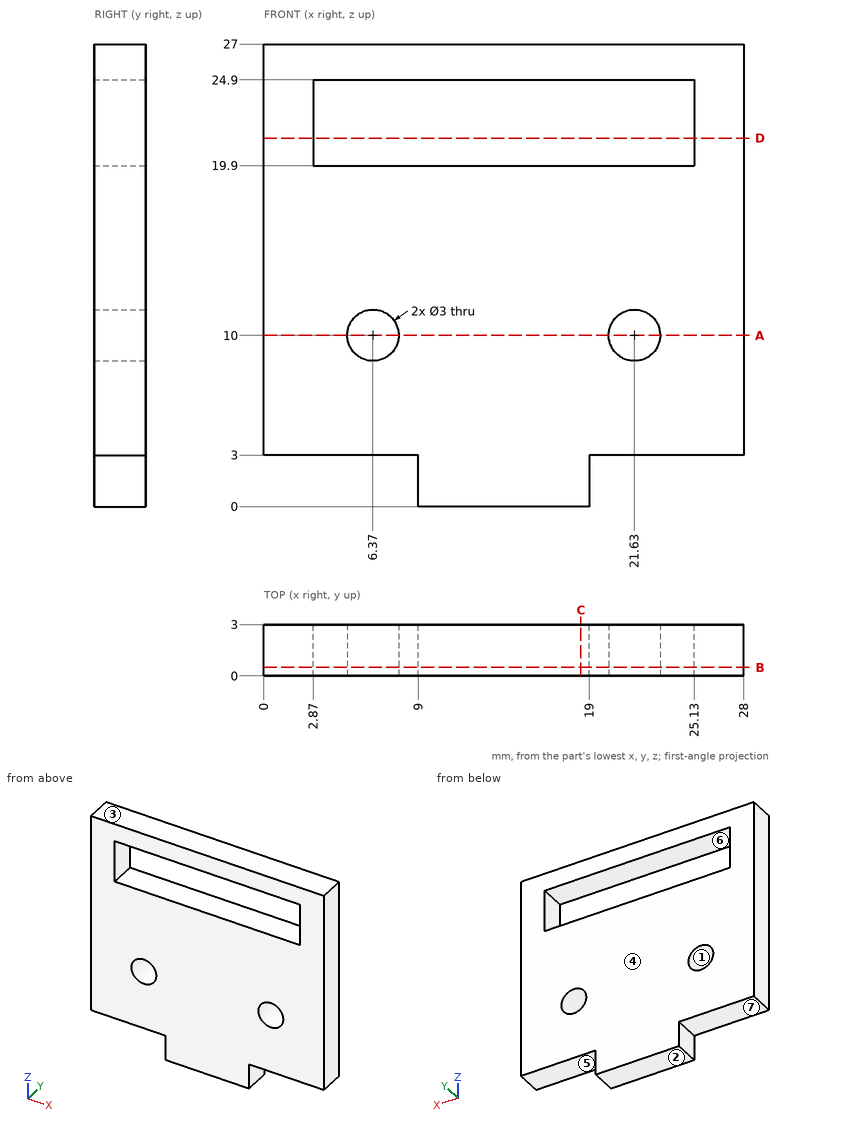
Job drawing, mm, ordinate dimensions from the low corner. One solid piece. A direction names the side the tool comes from. Give positions to 0.01 mm unless a question says otherwise; leave off trailing zeros. Order: outer loops, then holes, each group sorted by start corner. A loop starts at its lowest first (then second) coordinate and runs counter-clockwise, first axis right, second up. Notation, with made-up numbers: M 51.25,-24 L 79.25,-24 A33 ccw 79.25,6 Z; hole C 51.5,81 d4. An arc over 180 degrees is marked long. Put each result on its own line as item: value. Start each with the question number.
(1) Pull direction Z, two halves, no side cores. Call the marked faces 1, 2, 3 and 4: released by +Z, released by -Z, zero draft, split by the parting line, or undercut.
(2) Tool access for the marked faces 5, 6 and 7: list every direction of +Z, -Z, +X, -X, +Y, -Y with a clear straight run to the whole face (end or side of a thin tool).
(3) Band-saw the part on D-D on z = 21.5. Give the cut face in (x, y).
(4) Band-saw the part on B-B on y = 0.5. Give the cut face in (x, z), then the cut area to 3 significant figures.
(5) Drill centre lines: L1, parallel to X at y = 0.7, z = 10; L2, parallel to Z at x = 6.37, y = 0.9; L3, parallel to Z at x = 11.25, y = 0.2. Where is each one in solid material? Low to high. Write a range as [from, to].
(6) Pin check, flat tips, straight feed: pin 1 Ø1.5 at (y, z) = (1, 1) entering from +X; pin 2 Ø0.9 at (x, y) = (22.5, 2) entering from -Z; pin 3 Ø0.9 at (y, z) = (2, 1.5) entering from -X; pin 4 Ø1.8 at (x, z) = (21.63, 10) entering from -Y. Stop position of each tip, or through.
(7) Band-saw the part on A-A on z = 10. Give the cut face in (x, y).
(8) Band-saw the part on C-C on x = 18.5. Give the cut face in (y, z).
Results below:
1. face 1: undercut
1. face 2: released by -Z
1. face 3: released by +Z
1. face 4: zero draft
2. face 5: -Z, +X, +Y, -Y
2. face 6: +Y, -Y
2. face 7: -Z, -X, +Y, -Y
3. outline: M 0,0 L 2.87,0 L 2.87,3 L 0,3 Z; M 25.13,0 L 28,0 L 28,3 L 25.13,3 Z
4. outline: M 0,3 L 9,3 L 9,0 L 19,0 L 19,3 L 28,3 L 28,27 L 0,27 Z; hole M 2.87,19.9 L 25.13,19.9 L 25.13,24.9 L 2.87,24.9 Z; hole C 6.37,10 d3; hole C 21.63,10 d3
4. area: 577 mm2
5. L1: x = [0, 4.87], [7.87, 20.13], [23.13, 28]
5. L2: z = [3, 8.5], [11.5, 19.9], [24.9, 27]
5. L3: z = [0, 19.9], [24.9, 27]
6. pin 1: stops at x = 19
6. pin 2: stops at z = 3
6. pin 3: stops at x = 9
6. pin 4: passes through
7. outline: M 0,0 L 4.87,0 L 4.87,3 L 0,3 Z; M 7.87,0 L 20.13,0 L 20.13,3 L 7.87,3 Z; M 23.13,0 L 28,0 L 28,3 L 23.13,3 Z
8. outline: M 0,0 L 3,0 L 3,19.9 L 0,19.9 Z; M 0,24.9 L 3,24.9 L 3,27 L 0,27 Z
